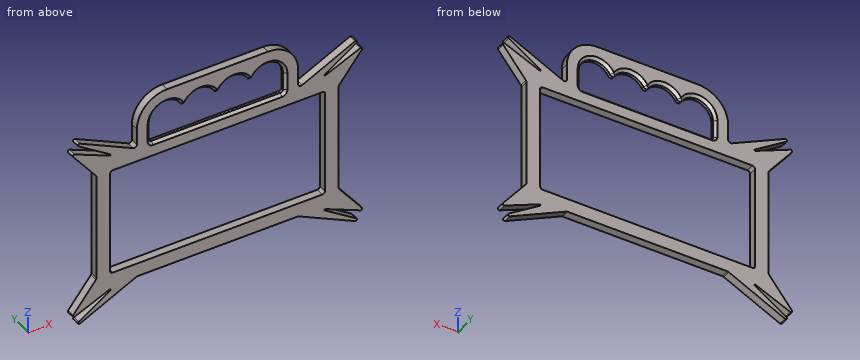
from build123d import *

# Parameters (mm, degrees)
F1_DEPTH = 6
F2_SIZE  = 1.99999


# Not quite as in the source:
# - a fillet or chamfer is up to 0.001 mm smaller than in the source, because OpenCascade refuses the exact size


with BuildPart() as f1:
    # F0 (on Front) → F1 (new body)
    with BuildSketch(Plane.XZ):
        with BuildLine():
            Line((-59.5457699822, -50), (59.5457699822, -50))
            ThreePointArc((59.5457699822, -50), (59.9887196894, -50.0496678342), (60.409669044, -50.1962044431))
            Line((60.409669044, -50.1962044431), (102.3891955872, -70.3016279512))
            ThreePointArc((102.3891955872, -70.3016279512), (103.6924020371, -69.8905574143), (103.3686877569, -68.5629523894))
            Line((103.3686877569, -68.5629523894), (79.7822069148, -53.1292204996))
            ThreePointArc((79.7822069148, -53.1292204996), (79.6153206959, -52.4745670657), (80.2529378835, -52.2512590929))
            Line((80.2529378835, -52.2512590929), (106.3328214803, -63.428352063))
            ThreePointArc((106.3328214803, -63.428352063), (107.5225378807, -63.1147703845), (107.5076095883, -61.8845119854))
            Line((107.5076095883, -61.8845119854), (90.4382623811, -40.5478279764))
            ThreePointArc((90.4382623811, -40.5478279764), (90.1127433617, -39.9604517642), (90, -39.2984378813))
            Line((90, -39.2984378813), (90, 39.2984378813))
            ThreePointArc((90, 39.2984378813), (90.1127433617, 39.9604517642), (90.4382623811, 40.5478279764))
            Line((90.4382623811, 40.5478279764), (107.5076095883, 61.8845119854))
            ThreePointArc((107.5076095883, 61.8845119854), (107.5225378807, 63.1147703845), (106.3328214803, 63.428352063))
            Line((106.3328214803, 63.428352063), (80.2529378835, 52.2512590929))
            ThreePointArc((80.2529378835, 52.2512590929), (79.6153206959, 52.4745670657), (79.7822069148, 53.1292204996))
            Line((79.7822069148, 53.1292204996), (103.3686877569, 68.5629523894))
            ThreePointArc((103.3686877569, 68.5629523894), (103.6924020371, 69.8905574143), (102.3891955872, 70.3016279512))
            Line((102.3891955872, 70.3016279512), (62.8638990618, 51.3716186976))
            ThreePointArc((62.8638990618, 51.3716186976), (60.9341196417, 51.4831084128), (60, 53.1754142545))
            Line((60, 53.1754142545), (60, 65))
            ThreePointArc((60, 65), (53.4099025767, 80.9099025767), (37.5, 87.5))
            Line((37.5, 87.5), (0, 87.5))
            Line((0, 87.5), (-37.5, 87.5))
            ThreePointArc((-37.5, 87.5), (-53.4099025767, 80.9099025767), (-60, 65))
            Line((-60, 65), (-60, 53.1754142545))
            ThreePointArc((-60, 53.1754142545), (-60.9341196417, 51.4831084128), (-62.8638990618, 51.3716186976))
            Line((-62.8638990618, 51.3716186976), (-102.3891955872, 70.3016279512))
            ThreePointArc((-102.3891955872, 70.3016279512), (-103.6924020371, 69.8905574143), (-103.3686877569, 68.5629523894))
            Line((-103.3686877569, 68.5629523894), (-79.7822069148, 53.1292204996))
            ThreePointArc((-79.7822069148, 53.1292204996), (-79.6153206959, 52.4745670657), (-80.2529378835, 52.2512590929))
            Line((-80.2529378835, 52.2512590929), (-106.3328214803, 63.428352063))
            ThreePointArc((-106.3328214803, 63.428352063), (-107.5225378807, 63.1147703845), (-107.5076095883, 61.8845119854))
            Line((-107.5076095883, 61.8845119854), (-90.4382623811, 40.5478279764))
            ThreePointArc((-90.4382623811, 40.5478279764), (-90.1127433617, 39.9604517642), (-90, 39.2984378813))
            Line((-90, 39.2984378813), (-90, -39.2984378813))
            ThreePointArc((-90, -39.2984378813), (-90.1127433617, -39.9604517642), (-90.4382623811, -40.5478279764))
            Line((-90.4382623811, -40.5478279764), (-107.5076095883, -61.8845119854))
            ThreePointArc((-107.5076095883, -61.8845119854), (-107.5225378807, -63.1147703845), (-106.3328214803, -63.428352063))
            Line((-106.3328214803, -63.428352063), (-80.2529378835, -52.2512590929))
            ThreePointArc((-80.2529378835, -52.2512590929), (-79.6153206959, -52.4745670657), (-79.7822069148, -53.1292204996))
            Line((-79.7822069148, -53.1292204996), (-103.3686877569, -68.5629523894))
            ThreePointArc((-103.3686877569, -68.5629523894), (-103.6924020371, -69.8905574143), (-102.3891955872, -70.3016279512))
            Line((-102.3891955872, -70.3016279512), (-60.409669044, -50.1962044431))
            ThreePointArc((-60.409669044, -50.1962044431), (-59.9887196894, -50.0496678342), (-59.5457699822, -50))
        make_face()
        with BuildLine():
            Line((-78, 40), (78, 40))
            ThreePointArc((78, 40), (79.4142135624, 39.4142135624), (80, 38))
            Line((80, 38), (80, -38))
            ThreePointArc((80, -38), (79.4142135624, -39.4142135624), (78, -40))
            Line((78, -40), (-78, -40))
            ThreePointArc((-78, -40), (-79.4142135624, -39.4142135624), (-80, -38))
            Line((-80, -38), (-80, 38))
            ThreePointArc((-80, 38), (-79.4142135624, 39.4142135624), (-78, 40))
        make_face(mode=Mode.SUBTRACT)
        with BuildLine():
            Line((48, 50), (40, 50))
            Line((40, 50), (0, 50))
            Line((0, 50), (-25, 50))
            Line((-25, 50), (-40, 50))
            Line((-40, 50), (-48, 50))
            ThreePointArc((-48, 50), (-49.4142135624, 50.5857864376), (-50, 52))
            Line((-50, 52), (-50, 65))
            ThreePointArc((-50, 65), (-40.7826608215, 77.0612660169), (-26.724137931, 71.3348872658))
            ThreePointArc((-26.724137931, 71.3348872658), (-25, 70.3484692283), (-23.275862069, 71.3348872658))
            ThreePointArc((-23.275862069, 71.3348872658), (-12.5, 77.5), (-1.724137931, 71.3348872658))
            ThreePointArc((-1.724137931, 71.3348872658), (0, 70.3484692283), (1.724137931, 71.3348872658))
            ThreePointArc((1.724137931, 71.3348872658), (12.5, 77.5), (23.275862069, 71.3348872658))
            ThreePointArc((23.275862069, 71.3348872658), (25, 70.3484692283), (26.724137931, 71.3348872658))
            ThreePointArc((26.724137931, 71.3348872658), (40.7826608215, 77.0612660169), (50, 65))
            Line((50, 65), (50, 52))
            ThreePointArc((50, 52), (49.4142135624, 50.5857864376), (48, 50))
        make_face(mode=Mode.SUBTRACT)
    extrude(amount=F1_DEPTH)

    # F2 (size 2 in the source; OpenCascade refuses exactly that, so slightly less here)
    f2_edges = [f1.edges().sort_by_distance(p)[0] for p in [
        (0, -6, 50),
        (0, 0, 50),
    ]]
    chamfer(f2_edges, length=F2_SIZE)


solid = f1.part
Build history of the part. All positions in model axes, mm. Coordinates: 2 decimals unless noted, no trailing zeros. Write each loop counter-clockwise with the first axis right and the second up, starting at its lowest first coordinate (ties: lowest second). Pieces come first, ordered by that corner, then holes.
(1) Drill centre lines: line 1 (Z direction, x = 12.5, y = -3.75); line 2 (X direction, y = -2, z = -10.5); line 3 (Z direction, x = -22.5, y = -3.75). Where is each one in solid material? Low to high.
(2) Pin check, flat tips, straight feed: pin 1 Ø3 at (y, z) = (-2.5, -18.5) entering from +X; pin 2 Ø1.8 at (x, y) = (27, -2.5) entering from -Z; pin 3 Ø1 at (y, z) = (-3, -43) entering from -X. Stop position of each tip, or through.
(3) Cut at C-C on z = -56.5. List the corners of the cut face in (x, y), and give its area (3 significant figures).
(4) Cut at A-A on z = -7.5. List the corners of the cut face in (x, y), and give its area (3 significant figures).
(5) Cut at D-D on x = -87.5. List the corners of the cut face in (y, z).
(6) Cut at B-B on x = -55.5. List the corners of the cut face in (y, z).
Working result:
1. line 1: z = -50 to -40, 40 to 50, 77.5 to 87.5
1. line 2: x = -90 to -80, 80 to 90
1. line 3: z = -50 to -40, 40 to 50, 72.5 to 87.5
2. pin 1: stops at x = 90
2. pin 2: stops at z = -50
2. pin 3: stops at x = -92.8
3. outline: (-103.2, -6) - (-90.17, -6) - (-90.17, 0) - (-103.2, 0) - close; (-84.93, -6) - (-73.57, -6) - (-73.57, 0) - (-84.93, 0) - close; (73.57, -6) - (84.93, -6) - (84.93, 0) - (73.57, 0) - close; (90.17, -6) - (103.2, -6) - (103.2, 0) - (90.17, 0) - close
3. area: 293 mm2
4. outline: (-90, -6) - (-80, -6) - (-80, 0) - (-90, 0) - close; (80, -6) - (90, -6) - (90, 0) - (80, 0) - close
4. area: 120 mm2
5. outline: (-6, -63.17) - (0, -63.17) - (0, -58.18) - (-6, -58.18) - close; (-6, -55.36) - (0, -55.36) - (0, 55.36) - (-6, 55.36) - close; (-6, 58.18) - (0, 58.18) - (0, 63.17) - (-6, 63.17) - close
6. outline: (-6, -50) - (0, -50) - (0, -40) - (-6, -40) - close; (-6, 40) - (0, 40) - (0, 78.5) - (-6, 78.5) - close
